```python
from build123d import *

# Parameters (mm, degrees)
BOSS_EXTRUDE1_DEPTH  = 79.375
M8_CLEARANCE_HOLE1_D = 9


with BuildPart() as part:
    # Sketch1 → Boss-Extrude1 (new, symmetric)
    with BuildSketch(Plane.XY):
        with BuildLine():
            Line((0, 0), (0, 31.75))
            ThreePointArc((0, 31.75), (3.367596045, 30.355096045), (4.7625, 26.9875))
            Line((4.7625, 26.9875), (4.7625, 9.525))
            ThreePointArc((4.7625, 9.525), (6.157403955, 6.157403955), (9.525, 4.7625))
            Line((9.525, 4.7625), (26.9875, 4.7625))
            ThreePointArc((26.9875, 4.7625), (30.355096045, 3.367596045), (31.75, 0))
            Line((31.75, 0), (0, 0))
        make_face()
    extrude(amount=BOSS_EXTRUDE1_DEPTH, both=True)

    # M8 Clearance Hole1 (through all)
    with Locations(Plane.ZY):
        with Locations((-57.15, 19.05), (57.15, 19.05)):
            Hole(M8_CLEARANCE_HOLE1_D / 2)


solid = part.part
```
Design review of the part built by this model. Coordinates are the model's own, in mm. A direction names the side the tool comes from. Coordinates: 2 decimals unless noted, no trailing zeros. Order: outer loops, then holes, each group sorted by start corner. A loop starts at its lowest first (then second) coordinate and runs counter-clockwise, first axis right, second up. Notation, with made-up numbers: (-10, 54) - (-2, 54) arc R34 ccw to (-2, 85) - close; hole circle Ø4 at (43.5, 26). An arc over 180 degrees is marked (long way). Answer in a Markdown table with one row per item.
(1) The part is to be moulded in two halves that separate along Z. For faces 3 (the cylindrical face through (3.33, 30.39, 1.11)), 4 (the flat face through (7, 5, 79.375)), 5 (the cylindrical face through (2.41, 23.51, -56.56)), 6 (the cylindrical face through (2.415, 19.248, 61.646)), say which applies: released by +Z, released by -Z, zero draft, split by the parting line, or undercut.
Checked values:
| item | result |
|---|---|
| face 3 | zero draft |
| face 4 | released by +Z |
| face 5 | undercut |
| face 6 | undercut |
(2) Wall thickness on line 1 along Z through (x, y) = (3, 19) (3 decimals); line 2 along Y through (x, z) = (10, 28): over which ranges is each line inside the solid? List them lowest first. Write a range as from..to.
Checked values:
| item | result |
|---|---|
| line 1 | -79.375..-61.65, -52.65..52.65, 61.65..79.375 |
| line 2 | 0..4.76 |
(3) Consider section D-D on y = 25. State the section outline as (x, z) points (1 decimal), plus the area to 3 significant figures.
Checked values:
| item | result |
|---|---|
| outline | (0, -79.4) - (4.8, -79.4) - (4.8, 79.4) - (0, 79.4) - close |
| area | 756 mm^2 |
(4) For faces 1 (the flat face through (4.762, 18, 1)), 2 (the flat face through (7, 5, -79.375)), list the 3-axis set-ups (+Z, -Z, +X, -X, +Y, -Y) from which the entire face can be reached by the end or side of a thin tool; tool diameter is ignored.
Checked values:
| item | result |
|---|---|
| face 1 | +Z, -Z, +X, +Y |
| face 2 | -Z, +X, -X, +Y, -Y |
(5) Clearance check with flat-ended pins moving along their axes: pin 1 (8.5 mm diameter, centred on x = 14.5, z = -6, fed in from +Y); pin 2 (14.5 mm diameter, centred on y = 19.05, z = 57.15, fed in from +X); pin 3 (2 mm diameter, centred on x = 28.5, z = 32, fed in from +Y); pin 4 (7 mm diameter, centred on y = 19.05, z = -57.15, fed in from -X). State where each tip first meets the part, or that it passes through.
Checked values:
| item | result |
|---|---|
| pin 1 | y = 4.76 |
| pin 2 | x = 4.76 |
| pin 3 | y = 4.73 |
| pin 4 | through |
(6) Consider section B-B on y = 19.05. Give the number of separate pieces and of enclosed holes in the cut face, plus the area to 3 significant figures.
Checked values:
| item | result |
|---|---|
| separate pieces | 3 |
| enclosed holes | 0 |
| area | 670 mm^2 |
